```python
from build123d import *

# Parameters (mm, degrees)
F0_W = 23.291029
F0_H = 14.848028


with BuildPart() as f1:
    # F0 (on Front) → F1 (revolve)
    with BuildSketch(Plane.XZ):
        Polygon((20.961925, 42.797264), (0, 42.797264), (0, 10.189825), (20.961925, 10.189825), (20.961925, 33.771988), align=None)
        Polygon((-43.961816, 10.189825), (-20.961925, 10.189825), (-20.961925, 33.771988), (-43.961816, 33.771988), (-43.961816, 25.037853), align=None)
        with Locations((-55.60733, 17.613839)):
            Rectangle(F0_W, F0_H)
        Polygon((0, 10.189825), (0, 42.797264), (-20.961925, 42.797264), (-20.961925, 33.771988), (-20.961925, 10.189825), align=None)
        Polygon((43.961816, 33.771988), (20.961925, 33.771988), (20.961925, 10.189825), (43.961816, 10.189825), (43.961816, 25.037853), align=None)
        with Locations((55.60733, 17.613839)):
            Rectangle(F0_W, F0_H)
    revolve(axis=Axis((-8.734133, 0, 0), (1, 0, 0)))


solid = f1.part
```
Input: part model. Units: mm. Frame: model coordinates. A direction names the side the tool comes from. Coordinates: 2 decimals unless noted, no trailing zeros. Loops run counter-clockwise (first coordinate to the right, second up) from the corner with the lowest first, then second, coordinate; pieces in that order, holes last. Notation, with made-up numbers: (60, 27.5) - (71, 27.5) arc R8 ccw to (71, 36.5) - close; hole circle Ø5 at (82.5, -9). An arc over 180 degrees is marked (long way). Answer in a Markdown table with one row per item.
(1) Mould query, pull axis Z, two halves, no side actions, for faces 4 (the face through (0.94, -3.06, 9.72)), 5 (the face through (-32.62, 20.55, -26.8)), 6 (the face through (-20.962, -13, 32)). Classes: pulls with the +Z half, pulls with the -Z half, needs draft (parallel to the pull), parting line crosses it, or undercut.
Model answer:
| item | result |
|---|---|
| face 4 | undercut |
| face 5 | parting line crosses it |
| face 6 | needs draft |
(2) Cut plane D-D on z = 23. Output: boundary loops of the cut face in (x, y), plus the area to 3 significant figures.
Model answer:
| item | result |
|---|---|
| outline | (-67.25, -9.89) - (-43.96, -9.89) - (-43.96, -24.73) - (-20.96, -24.73) - (-20.96, -36.09) - (20.96, -36.09) - (20.96, -24.73) - (43.96, -24.73) - (43.96, -9.89) - (67.25, -9.89) - (67.25, 9.89) - (43.96, 9.89) - (43.96, 24.73) - (20.96, 24.73) - (20.96, 36.09) - (-20.96, 36.09) - (-20.96, 24.73) - (-43.96, 24.73) - (-43.96, 9.89) - (-67.25, 9.89) - close |
| area | 6,220 mm² |
(3) Set-up query: faces 1 (the face through (-43.962, -0.2, -25.2)), 2 (the face through (32.3, 20.55, -26.8)), 3 (the face through (-0.29, 41.78, -9.28)). Return all of +Z, -Z, +X, -X, +Y, -Y with unobstructed straight access to the full face (end or side cutting, diameter ignored); none if empty.
Model answer:
| item | result |
|---|---|
| face 1 | -X |
| face 2 | +X |
| face 3 | +X, -X |
(4) Cut plane A-A on z = 0. Output: boundary loops of the cut face in (x, y).
Model answer:
| item | result |
|---|---|
| outline | (-67.25, -25.04) - (-43.96, -25.04) - (-43.96, -33.77) - (-20.96, -33.77) - (-20.96, -42.8) - (20.96, -42.8) - (20.96, -33.77) - (43.96, -33.77) - (43.96, -25.04) - (67.25, -25.04) - (67.25, -10.19) - (-67.25, -10.19) - close; (-67.25, 10.19) - (67.25, 10.19) - (67.25, 25.04) - (43.96, 25.04) - (43.96, 33.77) - (20.96, 33.77) - (20.96, 42.8) - (-20.96, 42.8) - (-20.96, 33.77) - (-43.96, 33.77) - (-43.96, 25.04) - (-67.25, 25.04) - close |
(5) Cut plane C-C on x = 55. Output: boundary loops of the cut face in (y, z), plus the area to 3 significant figures.
Model answer:
| item | result |
|---|---|
| outline | circle Ø50.08 at (0, 0); hole circle Ø20.38 at (0, 0) |
| area | 1,640 mm² |
(6) Material intervals for L1, parallel to Z at x = 20, y = 0; L2, parallel to Z at x = -21, y = 0, sorted ascending. Write a range as from..to.
Model answer:
| item | result |
|---|---|
| L1 | z = -42.8..-10.19, 10.19..42.8 |
| L2 | z = -33.77..-10.19, 10.19..33.77 |
(7) Pin query (flat end, axial travel): P1, Ø12, axis at y = -23.5, z = -22.5, coming from the -X side; P2, Ø1, axis at x = 6.5, z = 4, coming from the +Y side; P3, Ø6, axis at x = 42.5, y = -8.5, coming from the +Z side. Return the tip coordinate at first contact, or that it passes through.
Model answer:
| item | result |
|---|---|
| P1 | stops at x = -43.96 |
| P2 | stops at y = 42.65 |
| P3 | stops at z = 33.32 |
